```python
from build123d import *

# Parameters (mm, degrees)
F0_W     = 50
F0_H     = 80
F0_R     = 5
F0_R_2   = 8
F0_R_3   = 2.5
F1_DEPTH = 20
F2_START = 15
F2_DEPTH = 5


with BuildPart() as f1:
    # F0 (on Top) → F1 (new body)
    with BuildSketch(Plane.XY):
        Rectangle(F0_W, F0_H)
        with Locations((-15, -20)):
            Circle(F0_R, mode=Mode.SUBTRACT)
        with Locations((15, -20)):
            Circle(F0_R, mode=Mode.SUBTRACT)
        with Locations((-15, 20)):
            Circle(F0_R, mode=Mode.SUBTRACT)
        Circle(F0_R_2, mode=Mode.SUBTRACT)
        with Locations((15, 20)):
            Circle(F0_R, mode=Mode.SUBTRACT)
        with Locations((-15, 20)):
            Circle(F0_R)
        with Locations((-15, 20)):
            Circle(F0_R_3, mode=Mode.SUBTRACT)
        with Locations((15, 20)):
            Circle(F0_R)
        with Locations((15, 20)):
            Circle(F0_R_3, mode=Mode.SUBTRACT)
        with Locations((15, -20)):
            Circle(F0_R)
        with Locations((15, -20)):
            Circle(F0_R_3, mode=Mode.SUBTRACT)
        with Locations((-15, -20)):
            Circle(F0_R)
        with Locations((-15, -20)):
            Circle(F0_R_3, mode=Mode.SUBTRACT)
    extrude(amount=F1_DEPTH)

    # F0 (on Top) → F2 (cut)
    with BuildSketch(Plane.XY.offset(F2_START)):
        with Locations((-15, -20)):
            Circle(F0_R)
        with Locations((-15, -20)):
            Circle(F0_R_3, mode=Mode.SUBTRACT)
        with Locations((15, -20)):
            Circle(F0_R)
        with Locations((15, -20)):
            Circle(F0_R_3, mode=Mode.SUBTRACT)
        with Locations((-15, 20)):
            Circle(F0_R)
        with Locations((-15, 20)):
            Circle(F0_R_3, mode=Mode.SUBTRACT)
        with Locations((15, 20)):
            Circle(F0_R)
        with Locations((15, 20)):
            Circle(F0_R_3, mode=Mode.SUBTRACT)
    extrude(amount=F2_DEPTH, mode=Mode.SUBTRACT)


solid = f1.part
```
Can you work these out from the model? Positions are in its coordinate system, mm. A direction names the side the tool comes from. Coordinates: 2 decimals unless noted, no trailing zeros. Order: outer loops, then holes, each group sorted by start corner. A loop starts at its lowest first (then second) coordinate and runs counter-clockwise, first axis right, second up.
1. If we section it at B-B (z = 10.5): Please give me the cut outline in (x, y).
2. If we section it at C-C (y = -20): Please give me the cut outline in (x, z), then the cut area to 3 significant figures.
3. I need wall thicknesses on line 1 (Y direction, x = -15, z = 16.4); line 2 (Y direction, x = 12, z = 18); line 3 (Y direction, x = 0, z = 9.25). Which ranges of each line are inside material? Lowest first, please.
4. I'm going to push flat-ended pins straight in: pin 1 (5 mm diameter, centred on x = 14, y = 20, fed in from +Z); pin 2 (1.5 mm diameter, centred on x = 14.5, y = -19, fed in from +Z). Where does each tip first touch, or does it pass through?
5. For faces 5 (the face through (-1.73, -7.81, 9.86)), 6 (the face through (-16.08, -24.88, 17.46)), which set-ups out of +Z, -Z, +X, -X, +Y, -Y let a thin tool reach every point of the face, with its end or its side?
6. Thinking about a two-plate mould opening in X: for faces 1 (the face through (0, -40, 10)), 2 (the face through (25, -1, 10)), 3 (the face through (-25, -1, 10)), 4 (the face through (-16.84, -18.31, 7.4)), which applies, +X half, -X half, draft (parallel to the pull), parting line (faces both ways), or undercut?
7. If we section it at D-D (x = 0): Please give me the cut outline in (y, z), then the cut area to 3 significant figures.
8. If we section it at A-A (x = -15): Please give me the cut outline in (y, z).
Entries:
1. outline: (-25, -40) - (25, -40) - (25, 40) - (-25, 40) - close; hole circle Ø5 at (-15, -20); hole circle Ø5 at (-15, 20); hole circle Ø16 at (0, 0); hole circle Ø5 at (15, -20); hole circle Ø5 at (15, 20)
2. outline: (-25, 0) - (-17.5, 0) - (-17.5, 15) - (-20, 15) - (-20, 20) - (-25, 20) - close; (-12.5, 0) - (12.5, 0) - (12.5, 15) - (10, 15) - (10, 20) - (-10, 20) - (-10, 15) - (-12.5, 15) - close; (17.5, 0) - (25, 0) - (25, 20) - (20, 20) - (20, 15) - (17.5, 15) - close
2. area: 750 mm2
3. line 1: y = -40 to -25, -15 to 15, 25 to 40
3. line 2: y = -40 to -24, -16 to 16, 24 to 40
3. line 3: y = -40 to -8, 8 to 40
4. pin 1: stops at z = 15
4. pin 2: passes through
5. face 5: +Z, -Z
5. face 6: +Z
6. face 1: draft
6. face 2: +X half
6. face 3: -X half
6. face 4: undercut
7. outline: (-40, 0) - (-8, 0) - (-8, 20) - (-40, 20) - close; (8, 0) - (40, 0) - (40, 20) - (8, 20) - close
7. area: 1,280 mm2
8. outline: (-40, 0) - (-22.5, 0) - (-22.5, 15) - (-25, 15) - (-25, 20) - (-40, 20) - close; (-17.5, 0) - (17.5, 0) - (17.5, 15) - (15, 15) - (15, 20) - (-15, 20) - (-15, 15) - (-17.5, 15) - close; (22.5, 0) - (40, 0) - (40, 20) - (25, 20) - (25, 15) - (22.5, 15) - close
